Check sheet for the drawn part. Datum: minimum x, y, z corner. Units: mm. Round coordinates to 2 decimals unless told otherwise and drop trailing zeros. Write each loop counter-clockwise with the first axis right and the second up, starting at its lowest first coordinate (ties: lowest second). Pieces come first, ordered by that corner, then holes. Notation, with made-up numbers: (17.25, 72.25) -> (71.25, 72.25) arc R25 cw to (71.25, 103.25) -> close; hole circle Ø4 at (-21.75, 46). An arc over 180 degrees is marked (long way). Use CSV: the item, a comma, the result in double quotes.
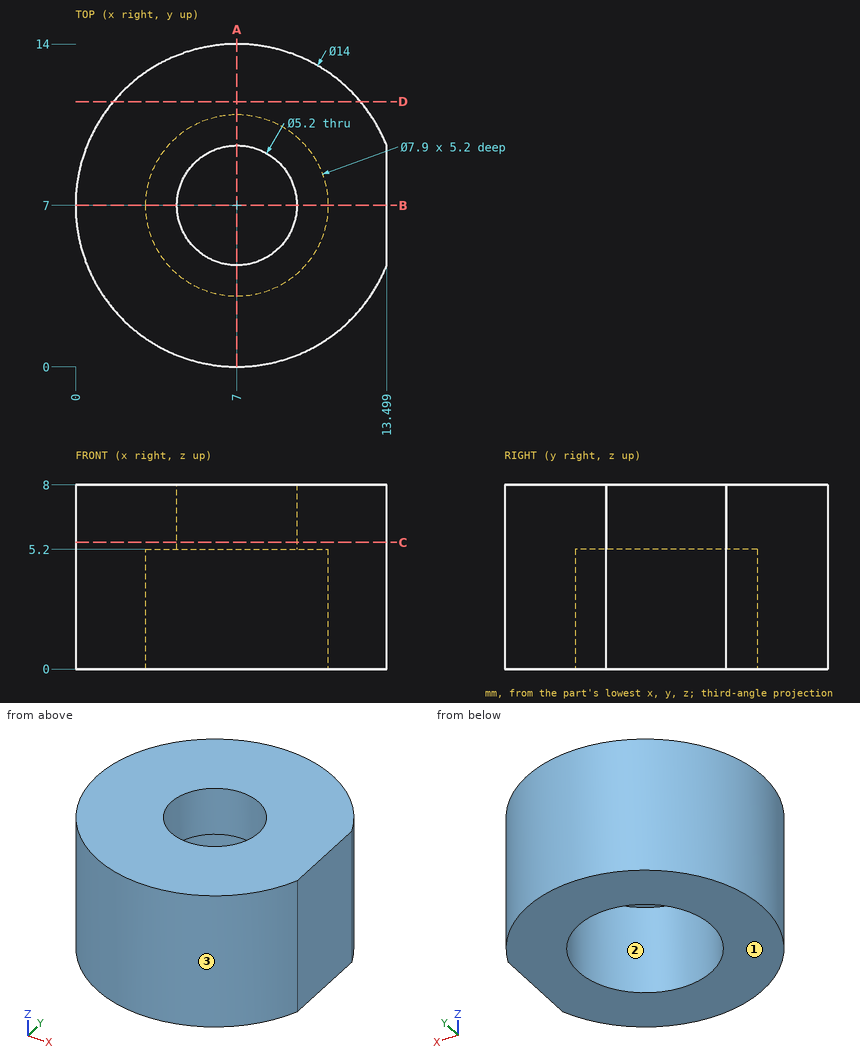
Q1. Section check C-C (z = 5.5). Record the cut outline in (x, y), plus the area to 3 significant figures.
Filled in:
outline,"(13.5, 4.4) -> (13.5, 9.6) arc R7 ccw (long way) to start; hole circle Ø5.2 at (7, 7)"
area,"131 mm²"
Q2. Section check B-B (y = 7). Record the cut outline in (x, z).
Filled in:
outline,"(0, 0) -> (3.05, 0) -> (3.05, 5.2) -> (4.4, 5.2) -> (4.4, 8) -> (0, 8) -> close; (9.6, 5.2) -> (10.95, 5.2) -> (10.95, 0) -> (13.5, 0) -> (13.5, 8) -> (9.6, 8) -> close"
Q3. Section check A-A (x = 7). Record the cut outline in (y, z).
Filled in:
outline,"(0, 0) -> (3.05, 0) -> (3.05, 5.2) -> (4.4, 5.2) -> (4.4, 8) -> (0, 8) -> close; (9.6, 5.2) -> (10.95, 5.2) -> (10.95, 0) -> (14, 0) -> (14, 8) -> (9.6, 8) -> close"
Q4. Material ranges on L1, parallel to Y at x = 7, z = 1.9; L2, parallel to Y at x = 7, z = 6.7; L3, parallel to X at y = 8, z = 4.5, recorded low to high.
Filled in:
L1,"0 to 3.05, 10.95 to 14"
L2,"0 to 4.4, 9.6 to 14"
L3,"0.07 to 3.18, 10.82 to 13.5"
Q5. Mould release check, pull along Y, two halves, no side actions. Record for the marked faces 1, 2 and 3: released by +Y, released by -Y, zero draft, split by the parting line, or undercut.
Filled in:
face 1,"zero draft"
face 2,"undercut"
face 3,"split by the parting line"
Q6. Go/stop test with flat-tipped pins: P1, Ø6.5, axis at x = 8, y = 7.5, coming from the -Z side; P2, Ø7, axis at x = 7, y = 7, coming from the -Z side; P3, Ø1.5, axis at x = 2, z = 4.5, coming from the -Y side; P4, Ø3, axis at x = 7, y = 7, coming from the +Z side. Record where each tip stops, or that it passes through.
Filled in:
P1,"z = 0"
P2,"z = 5.2"
P3,"y = 1.44"
P4,"through"
Q7. Section check D-D (y = 11.5). Record the cut outline in (x, z), plus the area to 3 significant figures.
Filled in:
outline,"(1.64, 0) -> (12.36, 0) -> (12.36, 8) -> (1.64, 8) -> close"
area,"85.8 mm²"
